from build123d import *

# Parameters (mm, degrees)
F1_DEPTH = 7.9375
F2_DEPTH = 7.9375
F0_W     = 57.15
F0_H     = 25.4
F3_DEPTH = 7.9375
F4_DEPTH = 7.9375
F5_DEPTH = 7.9375
F6_DEPTH = 7.9375
F0_W_2   = 88.9
F0_H_2   = 26.509378
F7_DEPTH = 7.9375


with BuildPart() as f1:
    # F0 (on Front) → F1 (new body, symmetric)
    with BuildSketch(Plane.XZ):
        Polygon((-232.758469, -69.13498), (-232.758469, -81.83498), (-105.758469, -81.83498), (-118.458469, -69.13498), align=None)
    extrude(amount=F1_DEPTH, both=True)

    # F0 (on Front) → F2 (join, symmetric)
    with BuildSketch(Plane.XZ):
        Polygon((-118.458469, -69.13498), (-105.758469, -81.83498), (-73.557188, -49.6337), (-73.557188, -24.2337), align=None)
    extrude(amount=F2_DEPTH, both=True)

    # F0 (on Front) → F3 (join, symmetric)
    with BuildSketch(Plane.XZ):
        with Locations((-44.982188, -36.9337)):
            Rectangle(F0_W, F0_H)
    extrude(amount=F3_DEPTH, both=True)

    # F0 (on Front) → F4 (join, symmetric)
    with BuildSketch(Plane.XZ):
        Polygon((-16.407188, -24.2337), (-16.407188, -49.6337), (15.794092, -81.83498), (28.494092, -69.13498), align=None)
    extrude(amount=F4_DEPTH, both=True)

    # F0 (on Front) → F5 (join, symmetric)
    with BuildSketch(Plane.XZ):
        Polygon((28.494092, -69.13498), (15.794092, -81.83498), (53.894092, -81.83498), (244.394092, -81.83498), (231.69601, -69.136898), (53.894092, -69.13498), align=None)
    extrude(amount=F5_DEPTH, both=True)

    # F0 (on Front) → F6 (join, symmetric)
    with BuildSketch(Plane.XZ):
        Polygon((231.69601, -69.136898), (244.394092, -81.83498), (276.599208, -50.743078), (276.599208, -24.2337), align=None)
    extrude(amount=F6_DEPTH, both=True)

    # F0 (on Front) → F7 (join, symmetric)
    with BuildSketch(Plane.XZ):
        with Locations((321.049208, -37.488389)):
            Rectangle(F0_W_2, F0_H_2)
    extrude(amount=F7_DEPTH, both=True)


solid = f1.part
Design review of the part built by this model. Coordinates are the model's own, in mm. A direction names the side the tool comes from. Round coordinates to 2 decimals unless told otherwise and drop trailing zeros. Write each loop counter-clockwise with the first axis right and the second up, starting at its lowest first coordinate (ties: lowest second). Pieces come first, ordered by that corner, then holes. Notation, with made-up numbers: M 50,64 L 99,64 A9 cw 99,79 Z; hole C 71,63 d10. An arc over 180 degrees is marked long. One line per item, written item: value. Start each with the question number.
1. Take a section at D-D on x = -167. State the section outline as (y, z) points, then the cut area to 3 significant figures.
2. For faces 1 (the face through (-45, 0, -49.634)), 2 (the face through (254.462, -0.111, -46.371)), 3 (the face through (-175, 0, -69.135)), list the 3-axis set-ups (+Z, -Z, +X, -X, +Y, -Y) from which the entire face can be reached by the end or side of a thin tool; tool diameter is ignored.
3. Take a section at B-B on z = -34. State the section outline as (x, y) points.
4. Take a section at A-A on y = -1.75. State the section outline as (x, z) points, then the cut area to 3 significant figures.
5. Take a section at C-C on z = -59. State the section outline as (x, y) points.
6. To check wall thickness, follow probe 1 along X at (y, z) = (-4.5, -60); probe 2 along X at (y, z) = (7, -64); probe 3 along Z at (x, y) = (106, 4.5). State the ranges of each line that lie inside material, in increasing order. Write a range as from..to.
7. Draft analysis for pull direction X (two halves, no side actions). For faces 4 (the face through (320, 0, -50.743)), 5 (the face through (-232.758, 0, -75)), 6 (the face through (-0.53, -0.11, -65.51)), state which applies: pulls with the +X half, pulls with the -X half, needs draft (parallel to the pull), parting line crosses it, or undercut.
8. Clearance check with flat-ended pins moving along their axes: P1, Ø2, axis at x = 212, y = -3, coming from the +Z side; P2, Ø12, axis at x = -115.5, z = -62, coming from the +Y side; P3, Ø2, axis at y = 5.5, z = -61, coming from the +X side; P4, Ø5, axis at x = 305, y = 0, coming from the -Z side. State where each tip first meets the part, or that it passes through.
Computed:
1. outline: M -7.94,-81.83 L 7.94,-81.83 L 7.94,-69.13 L -7.94,-69.13 Z
1. area: 202 mm²
2. face 1: -Z, +Y, -Y
2. face 2: +Z, +Y, -Y
2. face 3: +Z, -X, +Y, -Y
3. outline: M -83.32,-7.94 L -6.64,-7.94 L -6.64,7.94 L -83.32,7.94 Z; M 266.83,-7.94 L 365.5,-7.94 L 365.5,7.94 L 266.83,7.94 Z
4. outline: M -232.76,-81.83 L -105.76,-81.83 L -73.56,-49.63 L -16.41,-49.63 L 15.79,-81.83 L 244.39,-81.83 L 276.6,-50.74 L 365.5,-50.74 L 365.5,-24.23 L 276.6,-24.23 L 231.7,-69.14 L 53.89,-69.13 L 28.49,-69.13 L -16.41,-24.23 L -73.56,-24.23 L -118.46,-69.13 L -232.76,-69.13 Z
4. area: 11,000 mm²
5. outline: M -108.32,-7.94 L -82.92,-7.94 L -82.92,7.94 L -108.32,7.94 Z; M -7.04,-7.94 L 18.36,-7.94 L 18.36,7.94 L -7.04,7.94 Z; M 241.83,-7.94 L 268.05,-7.94 L 268.05,7.94 L 241.83,7.94 Z
6. probe 1: x = -109.32..-83.92, -6.04..19.36, 240.83..267.01
6. probe 2: x = -113.32..-87.92, -2.04..23.36, 236.83..262.87
6. probe 3: z = -81.83..-69.14
7. face 4: needs draft
7. face 5: pulls with the -X half
7. face 6: undercut
8. P1: stops at z = -69.14
8. P2: stops at y = 7.94
8. P3: stops at x = 267.01
8. P4: stops at z = -50.74
